Model file for the job. Use its own axes, mm. A direction names the side the tool comes from. Round coordinates to 2 decimals unless told otherwise and drop trailing zeros. Order: outer loops, then holes, each group sorted by start corner. A loop starts at its lowest first (then second) coordinate and runs counter-clockwise, first axis right, second up. Notation, with made-up numbers: (35, 13) -> (45, 13) arc R16 ccw to (45, 29) -> close; hole circle Ø11 at (40, 37.5). An arc over 180 degrees is marked (long way). Answer as CSV lines item,"result".
Autodesk Inventor part; units mm, degrees
ref_plane "YZ Plane" through (0, 0, 0) normal (1, 0, 0) x (0, 1, 0)
ref_plane "XZ Plane" through (0, 0, 0) normal (0, 1, 0) x (-1, 0, 0)
ref_plane "XY Plane" through (0, 0, 0) normal (0, 0, 1) x (1, 0, 0)
sketch "Sketch1" plane through (0, 0, 0) normal (0, 1, 0) x (-1, 0, 0)
  line L0 (0, 0) -> (24, 0)
  line L1 (24, 0) -> (24, -11)
  line L2 (24, -11) -> (0, -11)
  line L3 (0, -11) -> (0, 0)
  line L4 (24, -11) -> (35.6612, -11)
  line L5 (35.6612, -11) -> (35.6612, 0)
  line L6 (35.6612, 0) -> (24, 0)
  line L7 (24, 0) -> (24, -11)
  line L8 (0, 0) -> (0, 20)
  line L9 (0, -11) -> (0, -31)
  line L10 (0, -31) -> (-10, -31)
  line L11 (-10, -31) -> (-10, 20)
  line L12 (-10, 20) -> (0, 20)
  line L13 (35.6612, 0) -> (45.6612, 0)
  line L14 (45.6612, 0) -> (45.6612, 20)
  line L15 (45.6612, 20) -> (0, 20)
  line L16 (45.6612, 0) -> (45.6612, -31)
  line L17 (45.6612, -31) -> (0, -31)
  line L18 (39.1081, 4.4818) -> (-3.116, 4.4818)
  line L19 (-3.116, 4.4818) -> (-3.116, -14.9069)
  line L20 (-3.116, -14.9069) -> (39.1081, -14.9069)
  line L21 (39.1081, -14.9069) -> (39.1081, 4.4818)
  dimension "d0" = 24
  dimension "d1" = 11
  dimension "d2" = 20
  dimension "d3" = 20
  dimension "d4" = 10
  dimension "d6" = 10
extrude "Extrusion1" add sketch "Sketch1" along normal blind 15 contours L8 L18 L21 L13 L6 L0 | L3 L9 L20 L19 L18 L8 | L6 L5 L4 L1 | L2 L4 L5 L13 L21 L20 L9
extrude "Extrusion2" add sketch "Sketch1" along normal blind 5 contours L18 L19 L20 L9 L10 L11 L12 L8 | L8 L15 L14 L13 L21 L18 | L20 L21 L13 L16 L17 L9
fillet "Fillet1" radius 3.175 12 edges at (-17.8306, 5, 20) (10, 5, -5.5) (-17.8306, 5, -31) (-45.6612, 5, -5.5) (-17.996, 5, -14.9069) (-39.1081, 5, -5.2126) (-17.996, 5, 4.4818) (3.116, 5, -5.2126) (-39.1081, 10, -14.9069) (-39.1081, 10, 4.4818) (3.116, 10, -14.9069) (3.116, 10, 4.4818)
sketch "Sketch2" plane through (-45.6612, 0, -31) normal (-1, 0, 0) x (0, 0, 1)
  line L0 (51, 1.825) -> (0, 1.825)
  line L1 (20, 0) -> (31, 0)
  line L2 (23.2049, 1.825) -> (28.1129, 1.825)
  line L3 (28.1129, 1.825) -> (28.1129, 0)
  line L4 (28.1129, 0) -> (23.2049, 0)
  line L5 (23.2049, 0) -> (23.2049, 1.825)
extrude "Extrusion3" cut sketch "Sketch2" against normal blind 25
sketch "Sketch3" plane through (0, 15, 0) normal (0, 1, 0) x (1, 0, 0)
  line L0 (0, 0) -> (-24, 0)
  line L1 (-24, 11) -> (0, 11)
  line L2 (-24, 0) -> (-24, 11)
  line L3 (0, 11) -> (0, 0)
  line L4 (-24, 11) -> (0, 11)
  line L5 (0, 11) -> (0, 0)
  line L6 (0, 5.5) -> (2.5, 5.5)
  line L7 (-24, 2.8871) -> (-24, 7.7951)
  line L8 (-24, 5.3411) -> (-26.5, 5.3411)
  circle A0 centre (-26.5, 5.3411) radius 1
  dimension "d14" = 2.5
  dimension "d15" = 2.5
  dimension "d16" = 2
extrude "Extrusion4" cut sketch "Sketch3" against normal blind 2.5 contours A0
properties part number "turret x"
Q1. Saw through at D-D (y = 6.75). Write the cut outline in (x, z), plus the area to 3 significant figures.
Checks:
outline,"(-39.45, -11.73) arc R3.51 ccw to (-35.93, -15.24) -> (-0.06, -15.24) arc R3.51 ccw to (3.45, -11.73) -> (3.45, 1.31) arc R3.51 ccw to (-0.06, 4.82) -> (-35.93, 4.82) arc R3.51 ccw to (-39.45, 1.31) -> close; hole (-24, -11) -> (0, -11) -> (0, 0) -> (-24, 0) -> close"
area,"586 mm²"
Q2. Wall check: L1, parallel to Z at x = -26.5, y = 13.6; L2, parallel to Z at x = -2.5, y = 13.75; L3, parallel to Y at x = 6.5, z = -15. Give the ranges that are in metal, low to high. Write a range as [from, to].
Checks:
L1,"[-14.91, -6.34], [-4.34, 4.48]"
L2,"[-14.91, -11], [0, 4.48]"
L3,"[0, 5]"
Q3. Flat gauge pins, fed straight in: pin 1 (7.5 mm diameter, centred on x = -8.5, y = 8.5, fed in from +Z); pin 2 (9 mm diameter, centred on y = 5, z = -6, fed in from +X); pin 3 (6 mm diameter, centred on y = 9.5, z = -21.5, fed in from -X); pin 4 (1 mm diameter, centred on x = -24, y = 13, fed in from -Z). Where does each tip first touch, or does it go through?
Checks:
pin 1,"z = 18.06"
pin 2,"x = 10"
pin 3,"through"
pin 4,"z = -14.91"
Q4. Saw through at B-B (z = -20.5). Write the cut outline in (x, y) (3 decimals), plus the area to 3 significant figures.
Checks:
outline,"(-45.661, 0) -> (10, 0) -> (10, 1.825) arc R3.175 ccw to (6.825, 5) -> (-42.486, 5) arc R3.175 ccw to (-45.661, 1.825) -> close"
area,"274 mm²"
Q5. Saw through at A-A (x = -7.5). Write the cut outline in (y, z) (3 decimals), plus the area to 3 significant figures.
Checks:
outline,"(0, -31) -> (1.825, -31) arc R3.175 ccw to (5, -27.825) -> (5, -18.082) arc R3.175 cw to (8.175, -14.907) -> (15, -14.907) -> (15, -11) -> (0, -11) -> close; (0, 0) -> (15, 0) -> (15, 4.482) -> (8.175, 4.482) arc R3.175 cw to (5, 7.657) -> (5, 16.825) arc R3.175 ccw to (1.825, 20) -> (0, 20) -> close"
area,"284 mm²"
Q6. Saw through at C-C (x = -26.5). Write the cut outline in (y, z) (3 decimals), plus the area to 3 significant figures.
Checks:
outline,"(0, -31) -> (1.825, -31) arc R3.175 ccw to (5, -27.825) -> (5, -18.082) arc R3.175 cw to (8.175, -14.907) -> (15, -14.907) -> (15, -6.341) -> (12.5, -6.341) -> (12.5, -4.341) -> (15, -4.341) -> (15, 4.482) -> (8.175, 4.482) arc R3.175 cw to (5, 7.657) -> (5, 16.825) arc R3.175 ccw to (1.825, 20) -> (0, 20) -> (0, -2.887) -> (1.825, -2.887) -> (1.825, -7.795) -> (0, -7.795) -> close"
area,"435 mm²"
Q7. Tool access for faces 1 (the flat face through (-18, 12, -14.907)), 2 (the flat face through (-35, 1, -7.795)), 3 (the flat face through (-12, 7, 0)), 4 (the flat face through (-18, 12, 4.482)): list every direction of +Z, -Z, +X, -X, +Y, -Y with a clear straight run to the whole face (end or side of a thin tool).
Checks:
face 1,"-Z, +X, -X, +Y"
face 2,"-X, -Y"
face 3,"+Y, -Y"
face 4,"+Z, +X, -X, +Y"
Q8. Mould opens along Z. For faces 5 (the cylindrical face through (-17.44, 4.09, 19.05)), 6 (the flat face through (-27, 12.5, -5)), 7 (the cylindrical face through (-18.22, 4.09, -30.05)) say: +Z half, -Z half, draft (parallel to the pull), parting line (faces both ways), or undercut.
Checks:
face 5,"+Z half"
face 6,"undercut"
face 7,"-Z half"
